The figure shows three views and two pictorial views of one solid part (mm, origin at its lowest corner). Answer the questions. Round coordinates to 2 decimals unless told otherwise and drop trailing zeros. Order: outer loops, then holes, each group sorted by start corner. A loop starts at its lowest first (then second) coordinate and runs counter-clockwise, first axis right, second up. Notation, with made-up numbers: M 16.25,-37.5 L 67.25,-37.5 A24 ccw 67.25,-18.5 Z; hole C 11.25,-2 d8. An arc over 180 degrees is marked long. Return JSON: item names as keys, results as strings.
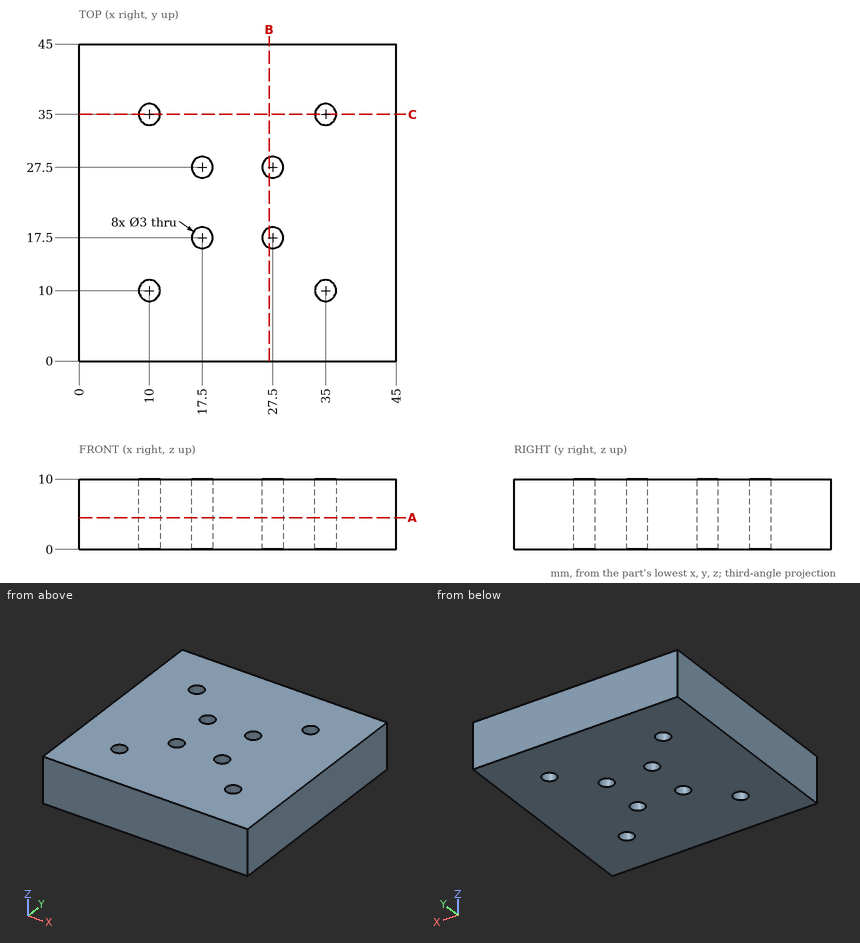
Item 1: Find section C-C (y = 35). Determine the outline of the cut face in (x, z).
Output:
{"outline": "M 0,0 L 8.5,0 L 8.5,10 L 0,10 Z; M 11.5,0 L 33.5,0 L 33.5,10 L 11.5,10 Z; M 36.5,0 L 45,0 L 45,10 L 36.5,10 Z"}
Item 2: Consider line 1 along Y through (x, z) = (17.5, 6.75); line 2 along Y through (x, z) = (35, 5.75); line 3 along X through (y, z) = (34, 4). Determine where each line is inside the solid, lowest interval first. Write a range as [from, to].
Output:
{"line 1": "y = [0, 16], [19, 26], [29, 45]", "line 2": "y = [0, 8.5], [11.5, 33.5], [36.5, 45]", "line 3": "x = [0, 8.88], [11.12, 33.88], [36.12, 45]"}
Item 3: Find section B-B (x = 27). Determine the outline of the cut face in (y, z), plus the area to 3 significant figures.
Output:
{"outline": "M 0,0 L 16.09,0 L 16.09,10 L 0,10 Z; M 18.91,0 L 26.09,0 L 26.09,10 L 18.91,10 Z; M 28.91,0 L 45,0 L 45,10 L 28.91,10 Z", "area": "393 mm^2"}
Item 4: Find section A-A (z = 4.5). State how many separate pieces and enclosed holes the cut face has, plus the area to 3 significant figures.
Output:
{"separate pieces": "1", "enclosed holes": "8", "area": "1,970 mm^2"}
